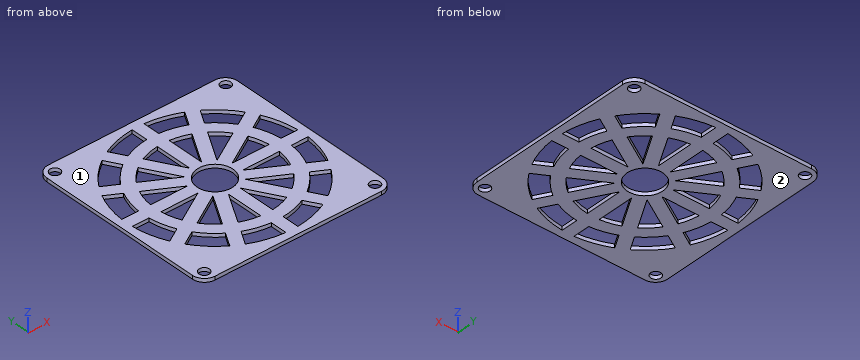
from build123d import *

# Parameters (mm, degrees)
F0_R     = 2.15
F2_DEPTH = 1.5
F1_R     = 30
F1_R_2   = 25
F3_DEPTH = 1.5
F4_R     = 7.5
F5_DEPTH = 25


with BuildPart() as f2:
    # F0 (on Top) → F2 (new body)
    with BuildSketch(Plane.XY):
        with BuildLine():
            ThreePointArc((40, 0), (28.2842712475, 28.2842712475), (0, 40))
            ThreePointArc((0, 40), (-28.2842712475, 28.2842712475), (-40, 0))
            ThreePointArc((-40, 0), (-28.2842712475, -28.2842712475), (0, -40))
            ThreePointArc((0, -40), (28.2842712475, -28.2842712475), (40, 0))
        make_face()
        with BuildLine():
            ThreePointArc((36.9154439226, 2.5), (36.9788549386, 1.2507147687), (37, 0))
            ThreePointArc((37, 0), (36.9788549386, -1.2507147687), (36.9154439226, -2.5))
            ThreePointArc((36.9154439226, -2.5), (35.7392555727, -9.5763046688), (33.2197122289, -16.2926584518))
            ThreePointArc((33.2197122289, -16.2926584518), (32.04293994, -18.5), (30.7197122289, -20.6227854707))
            ThreePointArc((30.7197122289, -20.6227854707), (26.1629509039, -26.1629509039), (20.6227854707, -30.7197122289))
            ThreePointArc((20.6227854707, -30.7197122289), (18.5, -32.04293994), (16.2926584518, -33.2197122289))
            ThreePointArc((16.2926584518, -33.2197122289), (9.5763046688, -35.7392555727), (2.5, -36.9154439226))
            ThreePointArc((2.5, -36.9154439226), (0, -37), (-2.5, -36.9154439226))
            ThreePointArc((-2.5, -36.9154439226), (-9.5763046688, -35.7392555727), (-16.2926584518, -33.2197122289))
            ThreePointArc((-16.2926584518, -33.2197122289), (-18.5, -32.04293994), (-20.6227854707, -30.7197122289))
            ThreePointArc((-20.6227854707, -30.7197122289), (-26.1629509039, -26.1629509039), (-30.7197122289, -20.6227854707))
            ThreePointArc((-30.7197122289, -20.6227854707), (-32.04293994, -18.5), (-33.2197122289, -16.2926584518))
            ThreePointArc((-33.2197122289, -16.2926584518), (-35.7392555727, -9.5763046688), (-36.9154439226, -2.5))
            ThreePointArc((-36.9154439226, -2.5), (-37, 0), (-36.9154439226, 2.5))
            ThreePointArc((-36.9154439226, 2.5), (-35.7392555727, 9.5763046688), (-33.2197122289, 16.2926584518))
            ThreePointArc((-33.2197122289, 16.2926584518), (-32.04293994, 18.5), (-30.7197122289, 20.6227854707))
            ThreePointArc((-30.7197122289, 20.6227854707), (-26.1629509039, 26.1629509039), (-20.6227854707, 30.7197122289))
            ThreePointArc((-20.6227854707, 30.7197122289), (-18.5, 32.04293994), (-16.2926584518, 33.2197122289))
            ThreePointArc((-16.2926584518, 33.2197122289), (-9.5763046688, 35.7392555727), (-2.5, 36.9154439226))
            ThreePointArc((-2.5, 36.9154439226), (0, 37), (2.5, 36.9154439226))
            ThreePointArc((2.5, 36.9154439226), (9.5763046688, 35.7392555727), (16.2926584518, 33.2197122289))
            ThreePointArc((16.2926584518, 33.2197122289), (18.5, 32.04293994), (20.6227854707, 30.7197122289))
            ThreePointArc((20.6227854707, 30.7197122289), (26.1629509039, 26.1629509039), (30.7197122289, 20.6227854707))
            ThreePointArc((30.7197122289, 20.6227854707), (32.04293994, 18.5), (33.2197122289, 16.2926584518))
            ThreePointArc((33.2197122289, 16.2926584518), (35.7392555727, 9.5763046688), (36.9154439226, 2.5))
        make_face(mode=Mode.SUBTRACT)
        with BuildLine():
            ThreePointArc((36.9154439226, -2.5), (36.9788549386, -1.2507147687), (37, 0))
            ThreePointArc((37, 0), (36.9788549386, 1.2507147687), (36.9154439226, 2.5))
            Line((36.9154439226, 2.5), (9.3301270189, 2.5))
            Line((9.3301270189, 2.5), (33.2197122289, 16.2926584518))
            ThreePointArc((33.2197122289, 16.2926584518), (32.04293994, 18.5), (30.7197122289, 20.6227854707))
            Line((30.7197122289, 20.6227854707), (6.8301270189, 6.8301270189))
            Line((6.8301270189, 6.8301270189), (20.6227854707, 30.7197122289))
            ThreePointArc((20.6227854707, 30.7197122289), (18.5, 32.04293994), (16.2926584518, 33.2197122289))
            Line((16.2926584518, 33.2197122289), (2.5, 9.3301270189))
            Line((2.5, 9.3301270189), (2.5, 36.9154439226))
            ThreePointArc((2.5, 36.9154439226), (0, 37), (-2.5, 36.9154439226))
            Line((-2.5, 36.9154439226), (-2.5, 9.3301270189))
            Line((-2.5, 9.3301270189), (-16.2926584518, 33.2197122289))
            ThreePointArc((-16.2926584518, 33.2197122289), (-18.5, 32.04293994), (-20.6227854707, 30.7197122289))
            Line((-20.6227854707, 30.7197122289), (-6.8301270189, 6.8301270189))
            Line((-6.8301270189, 6.8301270189), (-30.7197122289, 20.6227854707))
            ThreePointArc((-30.7197122289, 20.6227854707), (-32.04293994, 18.5), (-33.2197122289, 16.2926584518))
            Line((-33.2197122289, 16.2926584518), (-9.3301270183, 2.5))
            Line((-9.3301270183, 2.5), (-36.9154439226, 2.5))
            ThreePointArc((-36.9154439226, 2.5), (-37, 0), (-36.9154439226, -2.5))
            Line((-36.9154439226, -2.5), (-9.3301270189, -2.5))
            Line((-9.3301270189, -2.5), (-33.2197122289, -16.2926584518))
            ThreePointArc((-33.2197122289, -16.2926584518), (-32.04293994, -18.5), (-30.7197122289, -20.6227854707))
            Line((-30.7197122289, -20.6227854707), (-6.8301270191, -6.830127019))
            Line((-6.8301270191, -6.830127019), (-20.6227854707, -30.7197122289))
            ThreePointArc((-20.6227854707, -30.7197122289), (-18.5, -32.04293994), (-16.2926584518, -33.2197122289))
            Line((-16.2926584518, -33.2197122289), (-2.5, -9.3301270189))
            Line((-2.5, -9.3301270189), (-2.5, -36.9154439226))
            ThreePointArc((-2.5, -36.9154439226), (0, -37), (2.5, -36.9154439226))
            Line((2.5, -36.9154439226), (2.5, -9.3301270189))
            Line((2.5, -9.3301270189), (16.2926584518, -33.2197122289))
            ThreePointArc((16.2926584518, -33.2197122289), (18.5, -32.04293994), (20.6227854707, -30.7197122289))
            Line((20.6227854707, -30.7197122289), (6.8301270189, -6.8301270189))
            Line((6.8301270189, -6.8301270189), (30.7197122289, -20.6227854707))
            ThreePointArc((30.7197122289, -20.6227854707), (32.04293994, -18.5), (33.2197122289, -16.2926584518))
            Line((33.2197122289, -16.2926584518), (9.3301270189, -2.5))
            Line((9.3301270189, -2.5), (36.9154439226, -2.5))
        make_face()
        with BuildLine():
            Line((0, 40), (-35, 40))
            ThreePointArc((-35, 40), (-38.5355339059, 38.5355339059), (-40, 35))
            Line((-40, 35), (-40, 0))
            ThreePointArc((-40, 0), (-28.2842712475, 28.2842712475), (0, 40))
        make_face()
        with Locations((-35.85, 35.85)):
            Circle(F0_R, mode=Mode.SUBTRACT)
        with BuildLine():
            ThreePointArc((0, -40), (-28.2842712475, -28.2842712475), (-40, 0))
            Line((-40, 0), (-40, -35))
            ThreePointArc((-40, -35), (-38.5355339059, -38.5355339059), (-35, -40))
            Line((-35, -40), (0, -40))
        make_face()
        with Locations((-35.85, -35.85)):
            Circle(F0_R, mode=Mode.SUBTRACT)
        with BuildLine():
            Line((35, 40), (0, 40))
            ThreePointArc((0, 40), (28.2842712475, 28.2842712475), (40, 0))
            Line((40, 0), (40, 35))
            ThreePointArc((40, 35), (38.5355339059, 38.5355339059), (35, 40))
        make_face()
        with Locations((35.85, 35.85)):
            Circle(F0_R, mode=Mode.SUBTRACT)
        with BuildLine():
            Line((40, -35), (40, 0))
            ThreePointArc((40, 0), (28.2842712475, -28.2842712475), (0, -40))
            Line((0, -40), (35, -40))
            ThreePointArc((35, -40), (38.5355339059, -38.5355339059), (40, -35))
        make_face()
        with Locations((35.85, -35.85)):
            Circle(F0_R, mode=Mode.SUBTRACT)
    extrude(amount=F2_DEPTH)

    # F1 (on Top) → F3 (join)
    with BuildSketch(Plane.XY):
        Circle(F1_R)
        Circle(F1_R_2, mode=Mode.SUBTRACT)
    extrude(amount=F3_DEPTH)

    # F4 (on face) → F5 (cut)
    with BuildSketch(Plane.XY.offset(1.5)):
        Circle(F4_R)
    extrude(amount=-F5_DEPTH, mode=Mode.SUBTRACT)


solid = f2.part
Source: CAD feature listing. Evaluate the final solid. Frame: model axes, mm. Face numbers are marked on the shaded views. Give positions to 0.01 mm unless a question says otherwise; leave off trailing zeros. Order: outer loops, then holes, each group sorted by start corner. A loop starts at its lowest first (then second) coordinate and runs counter-clockwise, first axis right, second up. Notation, with made-up numbers: (79.25, 2) -> (118.25, 2) arc R33 cw to (118.25, 35) -> close; hole circle Ø7 at (49, 89.5). An arc over 180 degrees is marked (long way). Use a Markdown table: item, result.
1) Section query A-A, the plane x = 0. Return the cut outline in (y, z), then the cut area to 3 significant figures.
Answer list:
| item | result |
|---|---|
| outline | (-40, 0) -> (-7.5, 0) -> (-7.5, 1.5) -> (-40, 1.5) -> close; (7.5, 0) -> (40, 0) -> (40, 1.5) -> (7.5, 1.5) -> close |
| area | 97.5 mm² |
2) Ray query, line 1 along X through (y, z) = (-30, 0.8); line 2 along X through (y, z) = (-37, 0.85); line 3 along Y through (x, z) = (23, 1.2). Return the intervals inside material, ascending. Write a range as [from, to].
Answer list:
| item | result |
|---|---|
| line 1 | [-40, -21.66], [-20.21, -14.43], [-2.5, 2.5], [14.43, 20.21], [21.66, 40] |
| line 2 | [-39.58, -37.67], [-34.03, 34.03], [37.67, 39.58] |
| line 3 | [-40, -28.98], [-19.26, -9.8], [-2.5, 2.5], [9.8, 19.26], [28.98, 40] |
3) Mould query, pull axis Z, two halves, no side actions, for the marked faces 1 and 2. Classes: +Z half, -Z half, draft (parallel to the pull), parting line (faces both ways), or undercut.
Answer list:
| item | result |
|---|---|
| face 1 | +Z half |
| face 2 | -Z half |
4) Section query B-B, the plane z = 1.1. Count the separate pieces of the cut face and the enclosed holes in it, then the cut area to 3 significant figures.
Answer list:
| item | result |
|---|---|
| separate pieces | 1 |
| enclosed holes | 29 |
| area | 4,340 mm² |
